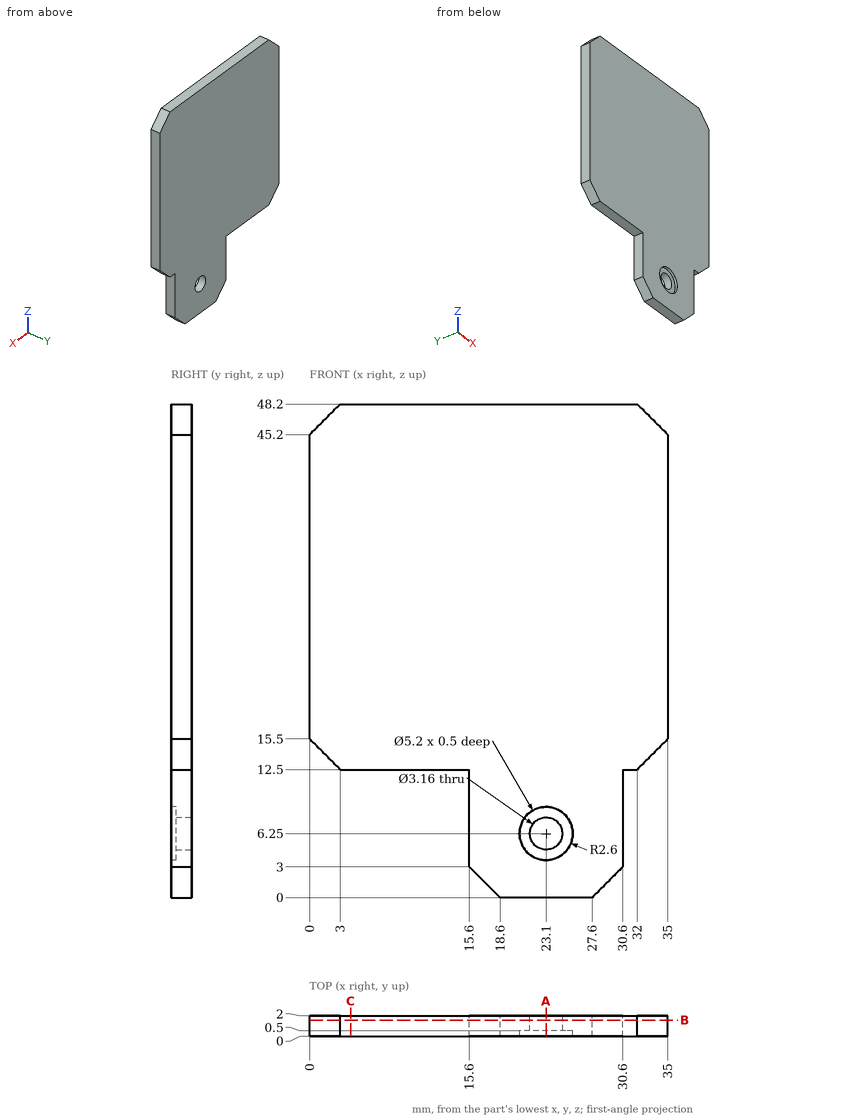
Part print with two shaded views. Sizes in mm from the minimum x, y, z corner. Round coordinates to 2 decimals unless told otherwise and drop trailing zeros. Loops run counter-clockwise (first coordinate to the right, second up) from the corner with the lowest first, then second, coordinate; pieces in that order, holes last. Notation, with made-up numbers: (79.25, 30) - (93.25, 30) arc R34 cw to (93.25, 66) - close; hole circle Ø9 at (-37, 59.5). An arc over 180 degrees is marked (long way). Put each result on its own line as item: value.
1. Slice it at B-B on y = 1.55. List the corners of the cut face in (x, z).
Geometry check:
outline: (0, 15.5) - (3, 12.5) - (15.6, 12.5) - (15.6, 3) - (18.6, 0) - (27.6, 0) - (30.6, 3) - (30.6, 12.5) - (32, 12.5) - (35, 15.5) - (35, 45.2) - (32, 48.2) - (3, 48.2) - (0, 45.2) - close; hole circle Ø3.16 at (23.1, 6.25)
2. Wall check: line 1 (X direction, y = 0.25, z = 6.25); line 2 (Z direction, x = 23.1, y = 0.2); line 3 (X direction, y = 1.7, z = 6.25). Give the ranges that are in metal, low to high.
Geometry check:
line 1: 15.6 to 20.5, 25.7 to 30.6
line 2: 0 to 3.65, 8.85 to 48.2
line 3: 15.6 to 21.52, 24.68 to 30.6
3. Pin check, flat tips, straight feed: P1, Ø4.5, axis at x = 23.1, z = 6.25, coming from the -Y side; P2, Ø0.6, axis at y = 1, z = 5.5, coming from the -X side; P3, Ø3, axis at x = 23.1, z = 6.25, coming from the -Y side; P4, Ø1.1, axis at x = 31, y = 0.5, coming from the -Z side. Stop position of each tip, or through.
Geometry check:
P1: y = 0.5
P2: x = 15.6
P3: through
P4: z = 2.85
4. Slice it at A-A on x = 23.1. List the corners of the cut face in (y, z).
Geometry check:
outline: (0, 0) - (2, 0) - (2, 4.67) - (0.5, 4.67) - (0.5, 3.65) - (0, 3.65) - close; (0, 8.85) - (0.5, 8.85) - (0.5, 7.83) - (2, 7.83) - (2, 48.2) - (0, 48.2) - close
5. Slice it at C-C on x = 4. List the corners of the cut face in (y, z), and give its area (3 significant figures).
Geometry check:
outline: (0, 12.5) - (2, 12.5) - (2, 48.2) - (0, 48.2) - close
area: 71.4 mm²
